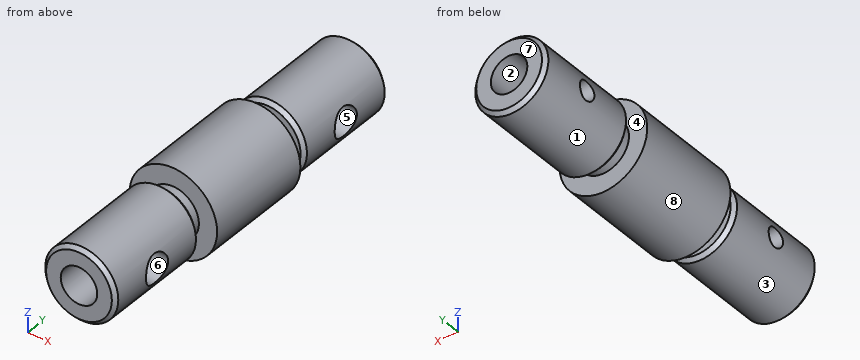
```python
from build123d import *

# Parameters (mm, degrees)
F0_R      = 5
F1_DEPTH  = 15
F2_R      = 3.5
F3_DEPTH  = 2
F4_R      = 6
F5_DEPTH  = 15
F6_R      = 3.5
F7_DEPTH  = 2
F8_R      = 5
F9_DEPTH  = 15
F10_SIZE  = 0.5
F12_R     = 1.3
F13_DEPTH = 25
F12_R_2   = 2
F14_DEPTH = 5
F15_R     = 2.5
F16_DEPTH = 50


with BuildPart() as f1:
    # F0 (on Front) → F1 (new body)
    with BuildSketch(Plane.XZ):
        Circle(F0_R)
    extrude(amount=F1_DEPTH)

    # F2 (on face) → F3 (join)
    with BuildSketch(Plane.XZ.offset(15)):
        Circle(F2_R)
    extrude(amount=F3_DEPTH)

    # F4 (on face) → F5 (join)
    with BuildSketch(Plane.XZ.offset(17)):
        Circle(F4_R)
    extrude(amount=F5_DEPTH)

    # F6 (on face) → F7 (join)
    with BuildSketch(Plane.XZ.offset(32)):
        Circle(F6_R)
    extrude(amount=F7_DEPTH)

    # F8 (on face) → F9 (join)
    with BuildSketch(Plane.XZ.offset(34)):
        Circle(F8_R)
    extrude(amount=F9_DEPTH)

    # F10
    f10_edges = [f1.edges().sort_by_distance(p)[0] for p in [
        (-5, -49, 0),
        (-5, -34, 0),
        (-5, 0, 0),
        (-5, -15, 0),
    ]]
    chamfer(f10_edges, length=F10_SIZE)

    # F12 (on offset) → F13 (cut)
    with BuildSketch(Plane.YZ.offset(5)):
        with Locations((-7.5, 0)):
            Circle(F12_R)
        with Locations((-41.5, 0)):
            Circle(F12_R)
    extrude(amount=-F13_DEPTH, mode=Mode.SUBTRACT)

    # F12 (on offset) → F14 (cut)
    with BuildSketch(Plane.YZ.offset(5)):
        with Locations((-41.5, 0)):
            Circle(F12_R_2)
        with Locations((-41.5, 0)):
            Circle(F12_R, mode=Mode.SUBTRACT)
        with Locations((-7.5, 0)):
            Circle(F12_R_2)
        with Locations((-7.5, 0)):
            Circle(F12_R, mode=Mode.SUBTRACT)
    extrude(amount=-F14_DEPTH, mode=Mode.SUBTRACT)

    # F15 (on face) → F16 (cut)
    with BuildSketch(Plane(origin=(0, 0, 0), x_dir=(-1, 0, 0), z_dir=(0, 1, 0))):
        Circle(F15_R)
    extrude(amount=-F16_DEPTH, mode=Mode.SUBTRACT)


solid = f1.part
```
Source: CAD feature listing. Evaluate the final solid. Frame: model axes, mm. Face numbers are marked on the shaded views. A direction names the side the tool comes from. Round coordinates to 2 decimals unless told otherwise and drop trailing zeros. Write each loop counter-clockwise with the first axis right and the second up, starting at its lowest first coordinate (ties: lowest second). Pieces come first, ordered by that corner, then holes. Notation, with made-up numbers: M 71,21 L 92,21 A11 cw 92,38 Z; hole C -5,41.25 d6. An arc over 180 degrees is marked long. Use CSV: the item, a comma, the result in double quotes. Start each with the question number.
Q1. Cut plane C-C on y = -15.5. Output: boundary loops of the cut face in (x, z), plus the area to 3 significant figures.
Q2. Line query: line 1 (Y direction, x = -2, z = 3.5); line 2 (Y direction, x = -2.75, z = 0); line 3 (Y direction, x = 3.7, z = 0). Output: solid intervals per line, ascending. Write a range as from..to.
Q3. First-contact query: P1, Ø3, axis at y = -19.5, z = -2, coming from the +X side; P2, Ø3.5, axis at y = -7.5, z = 0, coming from the +X side; P3, Ø5, axis at y = -41.5, z = 0, coming from the -X side. Flat tips, straight axial feed; report the tip coordinate or a pass-through.
Q4. Cut plane B-B on z = 0. Count the separate pieces of the cut face and the enclosed holes in it, plus the area to 3 significant figures.
Q5. Cut plane D-D on y = -41.5. Output: boundary loops of the cut face in (x, z).
Q6. Cut plane A-A on y = -7. Output: boundary loops of the cut face in (x, z).
Q7. Pull-direction query (Y, two-part tool) for the marked faces 5, 6, 7 and 8; classes: +Y half, -Y half, draft (parallel to the pull), parting line (faces both ways), or undercut.
Q8. Access query for the marked faces 1, 2, 3 and 4. Directions: +Z, -Z, +X, -X, +Y, -Y. A direction counts if a zero-diameter tool reaches every point of the face in a straight line with its end or side. Return the directions, or none.
Results found:
1,outline,"C 0,0 d7; hole C 0,0 d5"
1,area,"18.8 mm^2"
2,line 1,"-49..-34, -32..-17, -15..0"
2,line 2,"-49..-42.8, -40.2..-8.8, -6.2..0"
2,line 3,"-49..-43.5, -39.5..-34, -32..-17, -15..-9.5, -5.5..0"
3,P1,"x = 5.98"
3,P2,"x = -1.79"
3,P3,"x = -5"
4,separate pieces,"6"
4,enclosed holes,"0"
4,area,"229 mm^2"
5,outline,"M -4.83,-1.3 A5 ccw 4.58,-2 L 1.5,-2 A2.5 cw -2.14,-1.3 Z; M -4.83,1.3 L -2.14,1.3 A2.5 cw 1.5,2 L 4.58,2 A5 ccw Z"
6,outline,"M -4.85,-1.2 A5 ccw 4.61,-1.94 L 1.58,-1.94 A2.5 cw -2.19,-1.2 Z; M -4.85,1.2 L -2.19,1.2 A2.5 cw 1.58,1.94 L 4.61,1.94 A5 ccw Z"
7,face 5,"undercut"
7,face 6,"undercut"
7,face 7,"+Y half"
7,face 8,"draft"
8,face 1,"+Y"
8,face 2,"+Y, -Y"
8,face 3,"-Y"
8,face 4,"none"
